from build123d import *
from build123d.topology import SkipClean

# Parameters (mm, degrees)
SKETCH1_R           = 7.5
SKETCH1_R_2         = 2.5
BOSS_EXTRUDE1_DEPTH = 7
CUT_EXTRUDE2_REACH  = 14.708


with BuildPart() as part:
    # Sketch1 → Boss-Extrude1 (new body)
    with BuildSketch(Plane.XY):
        Circle(SKETCH1_R)
        Circle(SKETCH1_R_2, mode=Mode.SUBTRACT)
    extrude(amount=BOSS_EXTRUDE1_DEPTH)

    # Sketch2 → Cut-Revolve1 (revolve, cut)
    with BuildSketch(Plane(origin=(0, 0, 0), x_dir=(1, 0, 0), z_dir=(0, 1, 0)), mode=Mode.PRIVATE) as cut_revolve1_sk:
        Polygon((3, -4), (3, -3), (7.5, -1.5), (7.5, -5.5), align=None)
    revolve(cut_revolve1_sk.sketch.rotate(Axis((0, 0, 0), (0, 0, 1)), 180), axis=Axis((0, 0, 0), (0, 0, 1)), mode=Mode.SUBTRACT)

    # Cut-Extrude2: up to this cone (the profile starts outside it)
    with SkipClean():  # the faces are left unmerged after this step: merging them gives an invalid solid
        cut_extrude2_end = Plane(origin=(0, 0, 0), z_dir=(0, 0, 1)).offset(3.000001) * Cone(3e-06, 36.624, 12.207999, align=(Align.CENTER, Align.CENTER, Align.MIN), mode=Mode.PRIVATE)
        # Sketch3 → Cut-Extrude2 (cut, up to the surface)
        with BuildSketch(Plane.XY, mode=Mode.PRIVATE) as cut_extrude2_sk1:
            with BuildLine():
                Line((-0.768114575, -2.9), (0.768114575, -2.9))
                ThreePointArc((0.768114575, -2.9), (0, -3), (-0.768114575, -2.9))
            make_face()
        cut_extrude2_tool1 = extrude(cut_extrude2_sk1.sketch, amount=CUT_EXTRUDE2_REACH, mode=Mode.PRIVATE) - cut_extrude2_end
        add(cut_extrude2_tool1.solids().sort_by_distance((0, -2.940058, 0))[0], mode=Mode.SUBTRACT)


solid = part.part
For this review, take the finished solid that the model builds, in its own axes (mm). A direction names the side the tool comes from. Round coordinates to 2 decimals unless told otherwise and drop trailing zeros. Loops run counter-clockwise (first coordinate to the right, second up) from the corner with the lowest first, then second, coordinate; pieces in that order, holes last. Notation, with made-up numbers: (34, -30.75) - (55, -30.75) arc R31 cw to (55, -5.75) - close; hole circle Ø5 at (11, -16.75). An arc over 180 degrees is marked (long way). Put each result on its own line as item: value. Start each with the question number.
1. Consider section B-B on z = 4.75. State the section outline as (x, y) points.
2. For probe 1 along Z at (x, y) = (4.25, 2.25); probe 2 along Z at (x, y) = (-0.75, -5.25); probe 3 along Y at (x, z) = (0, 3.25), list the stretches that pass through material, from the lowest coordinate up. Write a range as [from, to].
3. Mouldability with a two-part tool opening along Y and no side actions: class faces 1 (the cylindrical face through (-7.493, 0.33, 0.74)), 2 (the cylindrical face through (-0.54, -2.44, 3.45)), 3 (the flat face through (-2, 2, 7)) as +Y half, -Y half, draft (parallel to the pull), parting line (faces both ways), or undercut.
4. Consider section A-A on y = 0. State the section outline as (x, z) points, plus the area to 3 significant figures.
5. Consider section D-D on z = 3.25. State the section outline as (x, y) points, plus the area to 3 significant figures.
6. For faces 4 (the cylindrical face through (0.1, 3, 3.5)), 5 (the cylindrical face through (-7.493, 0.33, 6.24)), list the 3-axis set-ups (+Z, -Z, +X, -X, +Y, -Y) from which the entire face can be reached by the end or side of a thin tool; tool diameter is ignored.
7. Consider section C-C on z = 6. State the section outline as (x, y) points.
8. Insertion check: P1, Ø2, axis at y = 5.5, z = 1.5, coming from the +X side. The pin has a flat end and moves straight along its axis. Give the tip position at first contact, or say it passes through.
Result sheet:
1. outline: circle Ø10.5 at (0, 0); hole circle Ø5 at (0, 0)
2. probe 1: [0, 2.4], [4.6, 7]
2. probe 2: [0, 2.23], [4.77, 7]
2. probe 3: [-2.9, -2.5], [2.5, 3]
3. face 1: parting line
3. face 2: undercut
3. face 3: draft
4. outline: (-7.5, 0) - (-2.5, 0) - (-2.5, 7) - (-7.5, 7) - (-7.5, 5.5) - (-3, 4) - (-3, 3) - (-7.5, 1.5) - close; (2.5, 0) - (7.5, 0) - (7.5, 1.5) - (3, 3) - (3, 4) - (7.5, 5.5) - (7.5, 7) - (2.5, 7) - close
4. area: 47.5 mm^2
5. outline: (-0.77, -2.9) - (0.77, -2.9) arc R3 ccw (long way) to start; hole circle Ø5 at (0, 0)
5. area: 8.54 mm^2
6. face 4: none
6. face 5: +Z, -Z
7. outline: circle Ø15 at (0, 0); hole circle Ø5 at (0, 0)
8. P1: x = 6
